Geometry: final body of the model. Coordinates: model frame, mm. Face numbers are marked on the shaded views. Round coordinates to 2 decimals unless told otherwise and drop trailing zeros. Order: outer loops, then holes, each group sorted by start corner. A loop starts at its lowest first (then second) coordinate and runs counter-clockwise, first axis right, second up. Notation, with made-up numbers: M -22.75,-10.5 L 21.25,-10.5 A29 cw 21.25,12.5 Z; hole C -22.5,47 d11. An arc over 180 degrees is marked long. Put each result on its own line as item: value. Start each with the question number.
1) First-contact query: P1, Ø4, axis at x = 5.625, z = -5.625, coming from the +Y side; P2, Ø3, axis at x = -2, z = 3.5, coming from the -Y side; P3, Ø2, axis at y = 5.5, z = -1, coming from the +X side. Flat tips, straight axial feed; report the tip coordinate or a pass-through.
2) Section B-B, the plane x = 0. Return loops of the section in (y, z), then the cut area to 3 significant figures.
3) Draft query along X for the marked faces 1, 2 and 3. Return one class per face: pulls with the +X half, pulls with the -X half, needs draft (parallel to the pull), parting line crosses it, or undercut.
4) Section C-C, the plane z = 6.75. Return loops of the section in (x, y), then the cut area to 3 significant figures.
5) Section A-A, the plane z = 0. Return loops of the section in (x, y).
6) Section D-D, the plane y = 2.5. Return loops of the section in (x, z), then the cut area to 3 significant figures.
7) Material intervals for probe 1 along X at (y, z) = (8.75, 0); probe 2 along Y at (x, z) = (-1, 6.75), sorted ascending. Write a range as [from, to].
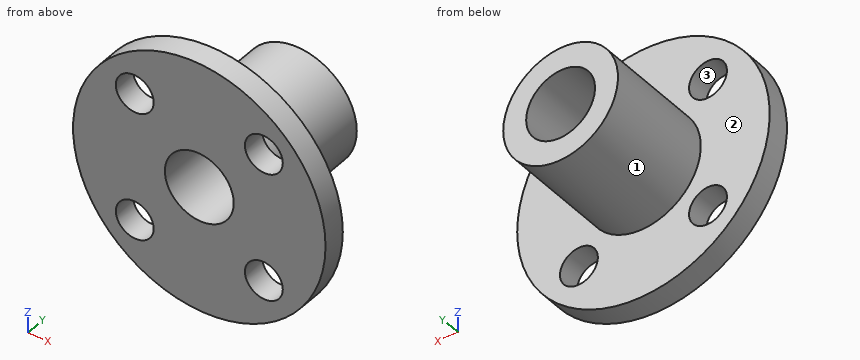
from build123d import *

# Parameters (mm, degrees)
SKETCH_3_R          = 1.65
CUT_EXTRUDE_1_DEPTH = 12.6


with BuildPart() as part:
    # 草图2 → 旋转1 (revolve)
    with BuildSketch(Plane.XY):
        Polygon((3, 11.6), (3, 0), (11, 0), (11, 2), (5, 2), (5, 11.6), align=None)
    revolve(axis=Axis((0, 0, 0), (0, 1, 0)))

    # 草图3 → 切除-拉伸1 (cut, through all)
    with BuildSketch(Plane.XZ):
        with Locations((-5.625, 5.625)):
            Circle(SKETCH_3_R)
        with Locations((5.625, 5.625)):
            Circle(SKETCH_3_R)
        with Locations((5.625, -5.625)):
            Circle(SKETCH_3_R)
        with Locations((-5.625, -5.625)):
            Circle(SKETCH_3_R)
    extrude(amount=-CUT_EXTRUDE_1_DEPTH, mode=Mode.SUBTRACT)


solid = part.part
Result sheet:
1. P1: stops at y = 2
1. P2: stops at y = 0
1. P3: stops at x = 5
2. outline: M 0,-11 L 2,-11 L 2,-5 L 11.6,-5 L 11.6,-3 L 0,-3 Z; M 0,3 L 11.6,3 L 11.6,5 L 2,5 L 2,11 L 0,11 Z
2. area: 70.4 mm2
3. face 1: parting line crosses it
3. face 2: needs draft
3. face 3: undercut
4. outline: M -8.69,0 L -6.83,0 L -6.83,2 L -8.69,2 Z; M -4.42,0 L 4.42,0 L 4.42,2 L -4.42,2 Z; M 6.83,0 L 8.69,0 L 8.69,2 L 6.83,2 Z
4. area: 25.1 mm2
5. outline: M -11,0 L -3,0 L -3,11.6 L -5,11.6 L -5,2 L -11,2 Z; M 3,0 L 11,0 L 11,2 L 5,2 L 5,11.6 L 3,11.6 Z
6. outline: C 0,0 d10; hole C 0,0 d6
6. area: 50.3 mm2
7. probe 1: x = [-5, -3], [3, 5]
7. probe 2: y = [0, 2]
